Verification items for the finished model (mm, model axes). Face numbers are marked on the shaded views. A direction names the side the tool comes from. Coordinates: 2 decimals unless noted, no trailing zeros. Loops run counter-clockwise (first coordinate to the right, second up) from the corner with the lowest first, then second, coordinate; pieces in that order, holes last. Notation, with made-up numbers: (38, 23.5) -> (94, 23.5) arc R16 cw to (94, 38.5) -> close; hole circle Ø4 at (-11.5, 16). An arc over 180 degrees is marked (long way). Answer as a JSON object with one key per item and string values. Group by question number.
Q1. Set-up check for the marked faces 1, 2 and 3: record each of +Z, -Z, +X, -X, +Y, -Y from which the full face is reachable in a straight line by a thin tool's end or side.
Q2. Scan lines: L1, parallel to Y at x = 0, z = 2.8; L2, parallel to Y at x = 0.5, z = 0.6; L3, parallel to X at y = 0.75, z = 2.8. Record each from-to range of solid material in increasing order.
Q3. Cross-section at B-B on z = 1.15. Record the boundary of the cut face in (x, y).
Q4. Gauge pin test, flat ends, axial feed: pin 1 Ø8 at (x, y) = (0, 0) entering from -Z; pin 2 Ø3.5 at (x, y) = (11, 0) entering from -Z; pin 3 Ø2.5 at (x, y) = (-11, 0) entering from +Z. Record the tip position at first contact, or that the pin passes through.
Q5. Cross-section at A-A on x = 0. Record the boundary of the cut face in (y, z), and give its area (3 significant figures).
Q6. Cross-section at C-C on y = -11. Record the boundary of the cut face in (x, z).
```python
from build123d import *

# Parameters (mm, degrees)
SKETCH_R        = 15
SKETCH_R_2      = 1.5
PAD_DEPTH       = 3
SKETCH002_R     = 2.5
POCKET_DEPTH    = 9
SKETCH001_R     = 5
POCKET001_DEPTH = 1
SKETCH003_R     = 2.5
POCKET002_DEPTH = 2


with BuildPart() as part:
    # Sketch → Pad (new body)
    with BuildSketch(Plane.XY):
        Circle(SKETCH_R)
        with Locations((0, 11)):
            Circle(SKETCH_R_2, mode=Mode.SUBTRACT)
        with Locations((-11, 0)):
            Circle(SKETCH_R_2, mode=Mode.SUBTRACT)
        with Locations((0, -11)):
            Circle(SKETCH_R_2, mode=Mode.SUBTRACT)
        with Locations((11, 0)):
            Circle(SKETCH_R_2, mode=Mode.SUBTRACT)
    extrude(amount=PAD_DEPTH)

    # Sketch002 (on Face7 of Pad) → Pocket (cut)
    with BuildSketch(Plane.XY.offset(3)):
        Circle(SKETCH002_R)
    extrude(amount=-POCKET_DEPTH, mode=Mode.SUBTRACT)

    # Sketch001 (on Face7 of Pad) → Pocket001 (cut)
    with BuildSketch(Plane.XY.offset(3)):
        Circle(SKETCH001_R)
    extrude(amount=-POCKET001_DEPTH, mode=Mode.SUBTRACT)

    # Sketch003 (on Face2 of Pocket001) → Pocket002 (cut)
    with BuildSketch(Plane(origin=(0, 0, 0), x_dir=(1, 0, 0), z_dir=(0, 0, -1))):
        with Locations((0, 11)):
            Circle(SKETCH003_R)
        with Locations((11, 0)):
            Circle(SKETCH003_R)
        with Locations((0, -11)):
            Circle(SKETCH003_R)
        with Locations((-11, 0)):
            Circle(SKETCH003_R)
    extrude(amount=-POCKET002_DEPTH, mode=Mode.SUBTRACT)


solid = part.part
```
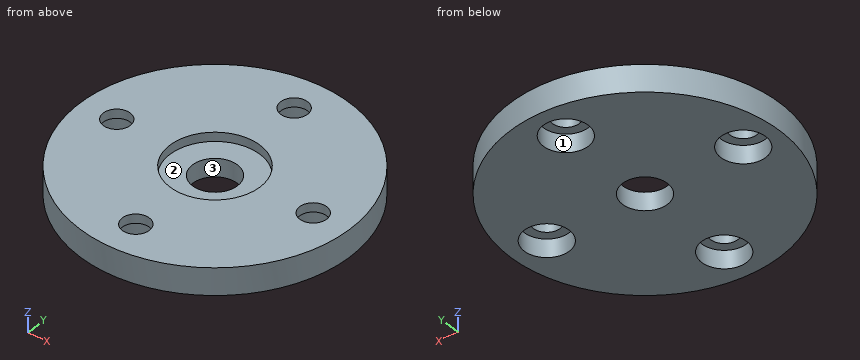
Computed values:
{
 "1": {"face 1": "-Z", "face 2": "+Z", "face 3": "+Z, -Z"},
 "2": {"L1": "y = -15 to -12.5, -9.5 to -5, 5 to 9.5, 12.5 to 15", "L2": "y = -14.99 to -13.45, -8.55 to -2.45, 2.45 to 8.55, 13.45 to 14.99", "L3": "x = -14.98 to -12.3, -9.7 to -4.94, 4.94 to 9.7, 12.3 to 14.98"},
 "3": {"outline": "circle Ø30 at (0, 0); hole circle Ø5 at (-11, 0); hole circle Ø5 at (0, -11); hole circle Ø5 at (0, 0); hole circle Ø5 at (0, 11); hole circle Ø5 at (11, 0)"},
 "4": {"pin 1": "stops at z = 0", "pin 2": "stops at z = 2", "pin 3": "passes through"},
 "5": {"outline": "(-15, 0) -> (-13.5, 0) -> (-13.5, 2) -> (-12.5, 2) -> (-12.5, 3) -> (-15, 3) -> close; (-9.5, 2) -> (-8.5, 2) -> (-8.5, 0) -> (-2.5, 0) -> (-2.5, 2) -> (-5, 2) -> (-5, 3) -> (-9.5, 3) -> close; (2.5, 0) -> (8.5, 0) -> (8.5, 2) -> (9.5, 2) -> (9.5, 3) -> (5, 3) -> (5, 2) -> (2.5, 2) -> close; (12.5, 2) -> (13.5, 2) -> (13.5, 0) -> (15, 0) -> (15, 3) -> (12.5, 3) -> close", "area": "44.0 mm²"},
 "6": {"outline": "(-10.2, 0) -> (-2.5, 0) -> (-2.5, 2) -> (-1.5, 2) -> (-1.5, 3) -> (-10.2, 3) -> close; (1.5, 2) -> (2.5, 2) -> (2.5, 0) -> (10.2, 0) -> (10.2, 3) -> (1.5, 3) -> close"}
}
